from build123d import *

# Parameters (mm, degrees)
SKETCH1_W               = 5
SKETCH1_H               = 110
BOSS_EXTRUDE1_DEPTH     = 3
BOSS_EXTRUDE2_DEPTH     = 55
BOSS_EXTRUDE3_START     = 55
BOSS_EXTRUDE3_DEPTH     = 55
SKETCH8_W               = 5
SKETCH8_H               = 10
BOSS_EXTRUDE4_DEPTH     = 3
SKETCH6_R               = 1.8
CUT_EXTRUDE1_DEPTH      = 66.117202028
SKETCH9_W               = 15
SKETCH9_H               = 110
BOSS_EXTRUDE5_DEPTH     = 3
FILLET1_R               = 1
CUT_EXTRUDE2_DEPTH      = 66.5
CUT_EXTRUDE2_DEPTH_BACK = 66.5
SKETCH10_R              = 1.8


with BuildPart() as part:
    # Sketch1 → Boss-Extrude1 (new body)
    with BuildSketch(Plane(origin=(0, 0, 0), x_dir=(1, 0, 0), z_dir=(0, 1, 0))):
        Rectangle(SKETCH1_W, SKETCH1_H)
    extrude(amount=BOSS_EXTRUDE1_DEPTH)

    # Sketch3 → Boss-Extrude2 (add)
    with BuildSketch(Plane.XY):
        with BuildLine():
            Line((-2.5, 3), (-2.5, 5.102989898))
            ThreePointArc((-2.5, 5.102989898), (0, 5.05), (2.5, 5.102989898))
            Line((2.5, 5.102989898), (2.5, 3))
            Line((2.5, 3), (2.5, 0))
            Line((2.5, 0), (-2.5, 0))
            Line((-2.5, 0), (-2.5, 3))
        make_face()
    extrude(amount=BOSS_EXTRUDE2_DEPTH)

    # Sketch7 → Boss-Extrude3 (add)
    with BuildSketch(Plane(origin=(0, 0, 0), x_dir=(-1, 0, 0), z_dir=(0, 0, -1)).offset(BOSS_EXTRUDE3_START)):
        with BuildLine():
            Line((-2.5, 5.102989898), (-2.5, 3))
            Line((-2.5, 3), (2.5, 3))
            Line((2.5, 3), (2.5, 5.102989898))
            ThreePointArc((2.5, 5.102989898), (0, 5.05), (-2.5, 5.102989898))
        make_face()
    extrude(amount=-BOSS_EXTRUDE3_DEPTH)

    # Sketch8 → Boss-Extrude4 (add)
    with BuildSketch(Plane.XZ):
        with Locations((0, 60)):
            Rectangle(SKETCH8_W, SKETCH8_H)
        with Locations((0, -60)):
            Rectangle(SKETCH8_W, SKETCH8_H)
    extrude(amount=-BOSS_EXTRUDE4_DEPTH)

    # Sketch6 → Cut-Extrude1 (cut, through all)
    with BuildSketch(Plane(origin=(0, 3, 0), x_dir=(1, 0, 0), z_dir=(0, 1, 0))):
        with Locations(Location((0, -62, 0), (0, 0, 270))):
            Circle(SKETCH6_R)
        with Locations(Location((0, 62, 0), (0, 0, 90))):
            Circle(SKETCH6_R)
    extrude(amount=-CUT_EXTRUDE1_DEPTH, mode=Mode.SUBTRACT)

    # Sketch9 → Boss-Extrude5 (add)
    with BuildSketch(Plane.XZ):
        Rectangle(SKETCH9_W, SKETCH9_H)
    extrude(amount=-BOSS_EXTRUDE5_DEPTH)

    # Fillet1
    # the kernel refuses this fillet: 1 mm, written as the material it adds along each edge
    with BuildSketch(Plane(origin=(2.5, 3, -55), x_dir=(0, 1, 0), z_dir=(0, 0, 1)), Plane(origin=(-2.5, 3, 55), x_dir=(0, 1, 0), z_dir=(0, 0, -1))) as fillet1_piece_1:
        with BuildLine():
            CenterArc((FILLET1_R, -FILLET1_R), FILLET1_R, 90, 90)
            Line((0, -FILLET1_R), (0, 0))
            Line((0, 0), (FILLET1_R, 0))
        make_face()
    extrude(amount=110)
    # the kernel refuses this fillet: 1 mm, written as the material it takes off along each edge
    with BuildSketch(Plane(origin=(-2.5, 5.102989898, 57.585592418), x_dir=(0, -1, 0), z_dir=(0, 0, -1))) as fillet1_2_piece_1:
        with BuildLine():
            CenterArc((1.034236967, -1), FILLET1_R, 90, 91.432543738)
            ThreePointArc((0.034549516, -1.025), (0.019501965, -0.512424928), (0, 0))
            Line((0, 0), (1.034236967, 0))
        make_face()
    extrude(amount=115.171184836, mode=Mode.SUBTRACT)
    with BuildSketch(Plane(origin=(2.5, 5.102989898, 57.585592418), x_dir=(0, -1, 0), z_dir=(0, 0, -1))) as fillet1_2_piece_2:
        with BuildLine():
            CenterArc((1.034236967, 1), FILLET1_R, 178.567456262, 91.432543738)
            ThreePointArc((0.034549516, 1.025), (0.019501965, 0.512424928), (0, 0))
            Line((0, 0), (1.034236967, 0))
        make_face()
    extrude(amount=115.171184836, mode=Mode.SUBTRACT)

    # Sketch10 → Cut-Extrude2 (cut, two sides: drawn at the far end of the back side and taken through both)
    with BuildSketch(Plane(origin=(0, 3, 0), x_dir=(1, 0, 0), z_dir=(0, 1, 0)).offset(-CUT_EXTRUDE2_DEPTH_BACK)):
        with Locations(Location((-3.75, -47.5, 0), (0, 0, 270))):
            Circle(SKETCH10_R)
        with Locations(Location((3.75, -41.5, 0), (0, 0, 270))):
            Circle(SKETCH10_R)
        with Locations(Location((3.75, 41.5, 0), (0, 0, 262.016443854))):
            Circle(SKETCH10_R)
        with Locations(Location((-3.75, 47.5, 0), (0, 0, 277.983556146))):
            Circle(SKETCH10_R)
    extrude(amount=CUT_EXTRUDE2_DEPTH + CUT_EXTRUDE2_DEPTH_BACK, mode=Mode.SUBTRACT)


solid = part.part
Read the model definition and answer for the solid it produces. Units are mm, in the model's axes. A direction names the side the tool comes from. Round coordinates to 2 decimals unless told otherwise and drop trailing zeros. Write each loop counter-clockwise with the first axis right and the second up, starting at its lowest first coordinate (ties: lowest second). Pieces come first, ordered by that corner, then holes. Notation, with made-up numbers: (-7.5, 73.5) - (18.5, 73.5) arc R19 cw to (18.5, 98.5) - close; hole circle Ø7 at (10, -6.5). An arc over 180 degrees is marked (long way). Use a Markdown table: item, result.
(1) Each of these flat-tipped pins is pushed along its axis until it touches: pin 1 Ø1.5 at (y, z) = (1.5, -60.5) entering from -X; pin 2 Ø1.2 at (x, z) = (-5, 8) entering from +Y; pin 3 Ø2.5 at (y, z) = (2, -60) entering from +X. Where does it stop, or does it pass through?
Reported:
| item | result |
|---|---|
| pin 1 | x = -2.5 |
| pin 2 | y = 3 |
| pin 3 | x = 2.5 |
(2) Straight lines are drawn through the part: line 1 along Z through (x, y) = (-0.25, 2.35); line 2 along Z through (x, y) = (3.5, 1.75); line 3 along X through (y, z) = (2.1, 62). For each, find the intervals that lie inside material, in ascending order. Write a range as [from, to].
Reported:
| item | result |
|---|---|
| line 1 | [-65, -63.78], [-60.22, 60.22], [63.78, 65] |
| line 2 | [-55, -43.28], [-39.72, 39.72], [43.28, 55] |
| line 3 | [-2.5, -1.8], [1.8, 2.5] |
(3) Which of the six approach directions +Z, -Z, +X, -X, +Y, -Y give full straight-line access (tool end or side, diameter ignored) to faces 5 (the flat face through (0, 3, -59)), 6 (the flat face through (-2.5, 1, 60)), 7 (the flat face through (-6, 3, 1))?
Reported:
| item | result |
|---|---|
| face 5 | -Z, +X, -X, +Y |
| face 6 | +Z, -X, +Y, -Y |
| face 7 | +Z, -Z, -X, +Y |
(4) The part is cut by section B-B (z = -47.5). Write down the section's boundary in (x, y) (3 decimals), then the cut area to 3 significant figures.
Reported:
| item | result |
|---|---|
| outline | (-7.5, 0) - (-5.55, 0) - (-5.55, 3) - (-7.5, 3) - close; (-1.95, 0) - (7.5, 0) - (7.5, 3) - (3.5, 3) arc R1 cw to (2.5, 4) - (2.5, 4.069) arc R1 ccw to (1.475, 5.068) arc R59 cw to (-1.475, 5.068) arc R1 ccw to (-1.95, 4.962) - close |
| area | 43.4 mm2 |
(5) The mould has two halves that part along Z. Classify faces 1 (the flat face through (2.5, 1, 60)), 2 (the cylindrical face through (-1.965, 1.895, 47.266)), 3 (the flat face through (0, 1, -65)), 4 (the cylindrical face through (-2.113, 1.895, -46.753)): released by +Z, released by -Z, zero draft, split by the parting line, or undercut.
Reported:
| item | result |
|---|---|
| face 1 | zero draft |
| face 2 | undercut |
| face 3 | released by -Z |
| face 4 | undercut |
(6) The part is cut by section A-A (x = 0). Write down the section's boundary in (y, z).
Reported:
| item | result |
|---|---|
| outline | (0, -65) - (3, -65) - (3, -63.8) - (0, -63.8) - close; (0, -60.2) - (3, -60.2) - (3, -55) - (5.05, -55) - (5.05, 55) - (3, 55) - (3, 60.2) - (0, 60.2) - close; (0, 63.8) - (3, 63.8) - (3, 65) - (0, 65) - close |
(7) The part is cut by section C-C (y = 1.8). Write down the section's boundary in (x, z).
Reported:
| item | result |
|---|---|
| outline | (-7.5, -55) - (-2.5, -55) - (-2.5, -65) - (2.5, -65) - (2.5, -55) - (7.5, -55) - (7.5, 55) - (2.5, 55) - (2.5, 65) - (-2.5, 65) - (-2.5, 55) - (-7.5, 55) - close; hole circle Ø3.6 at (-3.75, -47.5); hole circle Ø3.6 at (-3.75, 47.5); hole circle Ø3.6 at (0, -62); hole circle Ø3.6 at (0, 62); hole circle Ø3.6 at (3.75, -41.5); hole circle Ø3.6 at (3.75, 41.5) |
(8) The part is cut by section D-D (z = -62). Write down the section's boundary in (x, y), then the cut area to 3 significant figures.
Reported:
| item | result |
|---|---|
| outline | (-2.5, 0) - (-1.8, 0) - (-1.8, 3) - (-2.5, 3) - close; (1.8, 0) - (2.5, 0) - (2.5, 3) - (1.8, 3) - close |
| area | 4.20 mm2 |
